Geometry check sheet. Reference: the model listing, model coordinates, mm. Face numbers are marked on the shaded views. A direction names the side the tool comes from. Coordinates: 2 decimals unless noted, no trailing zeros. Loops run counter-clockwise (first coordinate to the right, second up) from the corner with the lowest first, then second, coordinate; pieces in that order, holes last.
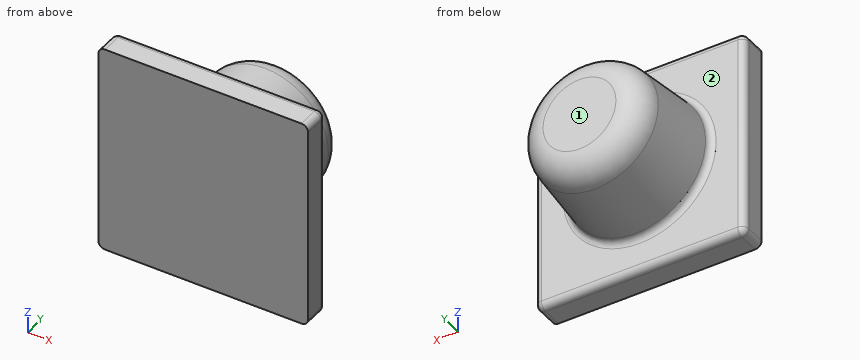
Autodesk Inventor part; units mm, degrees
ref_plane "YZ Plane" through (0, 0, 0) normal (1, 0, 0) x (0, 1, 0)
ref_plane "XZ Plane" through (0, 0, 0) normal (0, 1, 0) x (-1, 0, 0)
ref_plane "XY Plane" through (0, 0, 0) normal (0, 0, 1) x (1, 0, 0)
sketch "Sketch1" plane through (0, 0, 0) normal (1, 0, 0) x (0, 1, 0)
  line L0 (9, 0) -> (9, 4.5)
  line L1 (9, 4.5) -> (2, 5.2)
  line L2 (2, 5.2) -> (2, 7.2)
  line L3 (2, 7.2) -> (0, 7.2)
  line L4 (0, 7.2) -> (0, 0)
  line L5 (9, 0) -> (0, 0)
  dimension "d0" = 4.5
  dimension "d1" = 9
  dimension "d2" = 2
  dimension "d3" = 2
  dimension "d5" = 7.2
  dimension "d6" = 5.2
revolve "Revolution1" add sketch "Sketch1" angle 360 about axis through (0, 9, 0) along (0, -1, 0)
fillet "Fillet1" radius 2 1 edges at (0, 9, -4.5)
sketch "Sketch2" plane through (0, 0, 0) normal (0, -1, 0) x (1, 0, 0)
  line L0 (-7.75, -7.75) -> (7.75, -7.75)
  line L1 (7.75, -7.75) -> (7.75, 7.75)
  line L2 (7.75, 7.75) -> (-7.75, 7.75)
  line L3 (-7.75, 7.75) -> (-7.75, -7.75)
  line L4 (-7.75, -7.75) -> (7.75, 7.75) construction
  line L5 (7.75, -7.75) -> (-7.75, 7.75) construction
  point P0 (0, 0)
  dimension "d10" = 15.5
  dimension "d11" = 15.5
extrude "Extrusion1" add sketch "Sketch2" against normal up to surface (2 mm away)
fillet "Fillet4" radius 0.5 9 edges at (7.75, 1, 7.75) (0, 2, 7.75) (-7.75, 2, 0) (0, 2, -7.75) (7.75, 2, 0) (0, 2, -5.2) (7.75, 1, -7.75) (-7.75, 1, -7.75) (-7.75, 1, 7.75)
ref_plane "Work Plane1" through (0, 0, -7.25) normal (-1, 0, 0) x (0, 0, 1)
1) Section check A-A on z = 0. Record the cut outline in (x, y).
Data:
outline: (-7.75, 0) - (7.75, 0) - (7.75, 1.5) arc R0.5 ccw to (7.25, 2) - (5.65, 2) arc R0.5 cw to (5.15, 2.45) - (4.68, 7.2) arc R2 ccw to (2.69, 9) - (-2.69, 9) arc R2 ccw to (-4.68, 7.2) - (-5.15, 2.45) arc R0.5 cw to (-5.65, 2) - (-7.25, 2) arc R0.5 ccw to (-7.75, 1.5) - close
2) Material ranges on probe 1 along Y at (x, z) = (6.75, -4); probe 2 along Y at (x, z) = (-2.75, -0.25); probe 3 along X at (y, z) = (4.25, 2.75), recorded low to high.
Data:
probe 1: y = 0 to 2
probe 2: y = 0 to 9
probe 3: x = -4.15 to 4.15
3) Section check C-C on y = 5.5. Record the cut outline in (x, z).
Data:
outline: circle Ø9.7 at (0, 0)
4) Access from +Z, -Z, +X, -X, +Y, -Y to the whole of each face (thin tool, end or side, straight path). Record for the marked faces 1 and 2.
Data:
face 1: +Z, -Z, +X, -X, +Y
face 2: +Y
5) Depth check by flat-ended pin: pin 1 (3 mm diameter, centred on x = 5.5, z = -5, fed in from +Y); pin 2 (3 mm diameter, centred on x = 5, y = 5, fed in from -Z); pin 3 (5 mm diameter, centred on x = 4.5, z = 5.5, fed in from -Y). Enter the tip coordinate at first touch or a pass-through.
Data:
pin 1: stops at y = 2
pin 2: stops at z = -3.44
pin 3: stops at y = 0
6) Section check B-B on x = 0. Record the cut outline in (y, z).
Data:
outline: (0, -7.75) - (1.5, -7.75) arc R0.5 ccw to (2, -7.25) - (2, -5.65) arc R0.5 cw to (2.45, -5.15) - (7.2, -4.68) arc R2 ccw to (9, -2.69) - (9, 2.69) arc R2 ccw to (7.2, 4.68) - (2.45, 5.15) arc R0.5 cw to (2, 5.65) - (2, 7.25) arc R0.5 ccw to (1.5, 7.75) - (0, 7.75) - close
7) Section check D-D on x = -6. Record the cut outline in (y, z).
Data:
outline: (0, -7.75) - (1.5, -7.75) arc R0.5 ccw to (2, -7.25) - (2, 7.25) arc R0.5 ccw to (1.5, 7.75) - (0, 7.75) - close
